from build123d import *

# Parameters (mm, degrees)
SKETCH1_R                = 27.5
BOSS_EXTRUDE1_DEPTH      = 15
CHAMFER1_SIZE            = 2
SKETCH2_R                = 17.5
CUT_EXTRUDE1_DEPTH       = 12
SKETCH3_R                = 20.25
CUT_EXTRUDE2_DEPTH       = 3
SKETCH4_R                = 2
CUT_EXTRUDE3_DEPTH       = 42.683330001
BOSS_EXTRUDE2_DEPTH      = 9
SKETCH6_R                = 1.5
CUT_EXTRUDE4_DEPTH       = 41.700123015
CHAMFER2_SIZE            = 2
CHAMFER2_OF_MIRROR1_SIZE = 2
BOSS_EXTRUDE8_START      = 4.01
BOSS_EXTRUDE8_DEPTH      = 4.01
SKETCH14_W               = 23
SKETCH14_H               = 12
CUT_EXTRUDE5_DEPTH       = 10


with BuildPart() as part:
    # Sketch1 → Boss-Extrude1 (new body)
    with BuildSketch(Plane.XY):
        Circle(SKETCH1_R)
    extrude(amount=BOSS_EXTRUDE1_DEPTH)

    # Chamfer1
    chamfer1_edges = [part.edges().sort_by_distance(p)[0] for p in [
        (-27.5, 0, 15),
    ]]
    chamfer(chamfer1_edges, length=CHAMFER1_SIZE)

    # Sketch2 → Cut-Extrude1 (cut)
    with BuildSketch(Plane.XY.offset(15)):
        Circle(SKETCH2_R)
    extrude(amount=-CUT_EXTRUDE1_DEPTH, mode=Mode.SUBTRACT)

    # Sketch3 → Cut-Extrude2 (cut)
    with BuildSketch(Plane.XY.offset(15)):
        Circle(SKETCH3_R)
    extrude(amount=-CUT_EXTRUDE2_DEPTH, mode=Mode.SUBTRACT)

    # Sketch4 → Cut-Extrude3 (cut, through all)
    with BuildSketch(Plane(origin=(0, 0, 0), x_dir=(1, 0, 0), z_dir=(0, 1, 0))):
        with Locations(Location((0, -5, 0), (0, 0, 270))):
            Circle(SKETCH4_R)
    extrude(amount=-CUT_EXTRUDE3_DEPTH, mode=Mode.SUBTRACT)

    # Sketch5 → Boss-Extrude2 (add)
    with BuildSketch(Plane.XY.offset(12)):
        with BuildLine():
            ThreePointArc((-15.781356255, -1.926213803), (-14.875, 0), (-15.781356255, 1.926213803))
            ThreePointArc((-15.781356255, 1.926213803), (-16.724757779, 3.318673761), (-16.770509831, 5))
            ThreePointArc((-16.770509831, 5), (-17.5, 0), (-16.770509831, -5))
            ThreePointArc((-16.770509831, -5), (-16.724757779, -3.318673761), (-15.781356255, -1.926213803))
        make_face()
    boss_extrude2 = extrude(amount=-BOSS_EXTRUDE2_DEPTH)

    # Sketch6 → Cut-Extrude4 (cut, through all)
    with BuildSketch(Plane.XY.offset(12)):
        with Locations((-17.375, 0)):
            Circle(SKETCH6_R)
    cut_extrude4 = extrude(amount=-CUT_EXTRUDE4_DEPTH, mode=Mode.SUBTRACT)

    # Chamfer2
    chamfer2_edges = [part.edges().sort_by_distance(p)[0] for p in [
        (-18.875, 0, 0),
    ]]
    chamfer(chamfer2_edges, length=CHAMFER2_SIZE)

    # Mirror1: Boss-Extrude2, Cut-Extrude4 across plane
    add(boss_extrude2.mirror(Plane(origin=(0, 0, 0), x_dir=(0, 0, 1), z_dir=(1, 0, 0))))
    add(cut_extrude4.mirror(Plane(origin=(0, 0, 0), x_dir=(0, 0, 1), z_dir=(1, 0, 0))), mode=Mode.SUBTRACT)

    # Chamfer2 of Mirror1
    chamfer2_of_mirror1_edges = [part.edges().sort_by_distance(p)[0] for p in [
        (18.875, 0, 0),
    ]]
    chamfer(chamfer2_of_mirror1_edges, length=CHAMFER2_OF_MIRROR1_SIZE)

    # Sketch8 → Boss-Extrude8 (add)
    with BuildSketch(Plane.XY.offset(3).offset(BOSS_EXTRUDE8_START)):
        with BuildLine():
            Line((-2.696676707, -17.29097842), (-2.696676707, -9.629534503))
            ThreePointArc((-2.696676707, -9.629534503), (0.96452096, -9.953376277), (4.495419158, -8.932592378))
            Line((4.495419158, -8.932592378), (8.114072505, -15.505219359))
            ThreePointArc((8.114072505, -15.505219359), (2.852065596, -17.266027969), (-2.696676707, -17.29097842))
        make_face()
    extrude(amount=-BOSS_EXTRUDE8_DEPTH)

    # Sketch14 → Cut-Extrude5 (cut)
    with BuildSketch(Plane.XY.offset(12)):
        with Locations((0, 10.667708301)):
            Rectangle(SKETCH14_W, SKETCH14_H)
    extrude(amount=-CUT_EXTRUDE5_DEPTH, mode=Mode.SUBTRACT)


solid = part.part
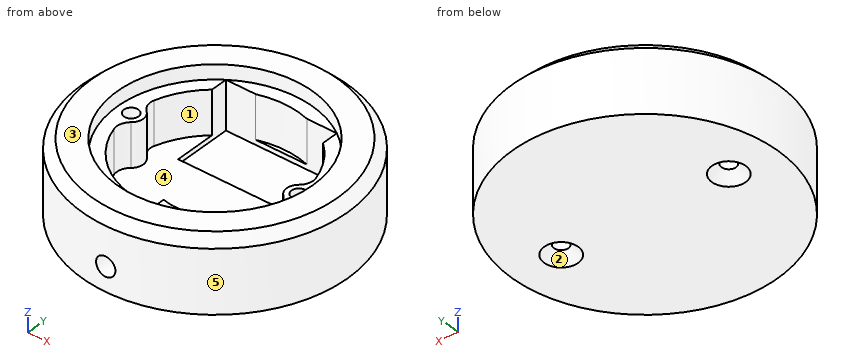
Read the model definition and answer for the solid it produces. Units are mm, in the model's axes. Face numbers are marked on the shaded views. A direction names the side the tool comes from. Give positions to 0.01 mm unless a question says otherwise; leave off trailing zeros. Write each loop counter-clockwise with the first axis right and the second up, starting at its lowest first coordinate (ties: lowest second). Pieces come first, ordered by that corner, then holes. Notation, with made-up numbers: (34.5, 52.25) -> (78.5, 52.25) arc R17 cw to (78.5, 73.25) -> close; hole circle Ø6 at (-24.75, -27.75). An arc over 180 degrees is marked (long way). Answer as a JSON object with one key per item and string values. Group by question number.
1) Find section C-C (z = 5). Write down the section's boundary in (x, y) (1 decimal), and give its area (3 significant figures).
2) Consider L1, parallel to Y at x = 0.5, z = 8.75; L2, parallel to Y at x = 0, z = 12.85; L3, parallel to Y at x = -16, z = 8.75. Determine where each line is inside the solid, lowest interval first. Write a range as from..to.
3) Find section B-B (z = 8.25). Write down the section's boundary in (x, y) (1 decimal).
4) The mould has two halves that part along X. Classify the marked faces 3, 4 and 5: +X half, -X half, draft (parallel to the pull), parting line (faces both ways), or undercut.
5) Each of these flat-tipped pins is pushed along its axis until it touches: P1, Ø6, axis at x = -11.5, z = 5, coming from the -Y side; P2, Ø7, axis at x = 1, y = -14, coming from the +Z side; P3, Ø4, axis at x = -2.5, z = 3, coming from the +Y side. Where does it stop, or does it pass through?
6) Find section A-A (y = 0). Write down the section's boundary in (x, z) (3 decimals).
7) A tool of negligible diameter and unlimited length cuts with its end or side. For the marked faces 1 and 2, from which of +Z, -Z, +X, -X, +Y, -Y can it reach the whole face along a straight path? Write none if from no direction.
Values follow:
{
 "1": {"outline": "(-2, -27.4) -> (-2, -17.4) arc R17.5 ccw to (2, -17.4) -> (2, -27.4) arc R27.5 ccw (long way) to start; hole circle Ø3 at (-17.4, 0); hole (-16.8, -5) arc R17.5 ccw to (-2.7, -17.3) -> (-2.7, -9.6) arc R10 ccw to (4.5, -8.9) -> (8.1, -15.5) arc R17.5 ccw to (16.8, -5) arc R3 ccw to (15.8, -1.9) arc R2.5 cw to (15.8, 1.9) arc R3 ccw to (16.8, 5) arc R17.5 ccw to (11.5, 13.2) -> (11.5, 16.7) -> (5.3, 16.7) arc R17.5 ccw to (-5.3, 16.7) -> (-11.5, 16.7) -> (-11.5, 13.2) arc R17.5 ccw to (-16.8, 5) arc R3 ccw to (-15.8, 1.9) arc R2.5 cw to (-15.8, -1.9) arc R3 ccw to start; hole circle Ø3 at (17.4, 0)", "area": "1,440 mm2"},
 "2": {"L1": "y = -27.5..-17.49, 17.49..27.5", "L2": "y = -27.5..-20.25, 20.25..27.5", "L3": "y = -22.37..-7.09, -2.13..-0.6, 0.6..2.13, 7.09..22.37"},
 "3": {"outline": "circle Ø55 at (0, 0); hole circle Ø3 at (-17.4, 0); hole (-16.8, -5) arc R17.5 ccw to (16.8, -5) arc R3 ccw to (15.8, -1.9) arc R2.5 cw to (15.8, 1.9) arc R3 ccw to (16.8, 5) arc R17.5 ccw to (11.5, 13.2) -> (11.5, 16.7) -> (5.3, 16.7) arc R17.5 ccw to (-5.3, 16.7) -> (-11.5, 16.7) -> (-11.5, 13.2) arc R17.5 ccw to (-16.8, 5) arc R3 ccw to (-15.8, 1.9) arc R2.5 cw to (-15.8, -1.9) arc R3 ccw to start; hole circle Ø3 at (17.4, 0)"},
 "4": {"face 3": "draft", "face 4": "undercut", "face 5": "parting line"},
 "5": {"P1": "stops at y = -26.15", "P2": "stops at z = 12", "P3": "stops at y = 27.5"},
 "6": {"outline": "(-27.5, 0) -> (-20.875, 0) -> (-18.875, 2) -> (-18.875, 12) -> (-20.25, 12) -> (-20.25, 15) -> (-25.5, 15) -> (-27.5, 13) -> close; (-15.875, 2) -> (-13.875, 0) -> (13.875, 0) -> (15.875, 2) -> (15.875, 12) -> (14.875, 12) -> (14.875, 3) -> (-14.875, 3) -> (-14.875, 12) -> (-15.875, 12) -> close; (18.875, 2) -> (20.875, 0) -> (27.5, 0) -> (27.5, 13) -> (25.5, 15) -> (20.25, 15) -> (20.25, 12) -> (18.875, 12) -> close"},
 "7": {"face 1": "+Z", "face 2": "-Z"}
}
